from build123d import *

# Parameters (mm, degrees)
SKETCH1_R           = 6.35
BOSS_EXTRUDE1_DEPTH = 31.75
CUT_EXTRUDE1_DEPTH  = 19.05
SKETCH3_R           = 3.175
CUT_EXTRUDE2_DEPTH  = 12.7


with BuildPart() as part:
    # Sketch1 → Boss-Extrude1 (new body)
    with BuildSketch(Plane.XY):
        Circle(SKETCH1_R)
    extrude(amount=BOSS_EXTRUDE1_DEPTH)

    # Sketch2 → Cut-Extrude1 (cut)
    with BuildSketch(Plane.XY.offset(31.75)):
        with BuildLine():
            Line((2.016062499, 2.286), (-2.016062499, 2.286))
            ThreePointArc((-2.016062499, 2.286), (0, -3.048), (2.016062499, 2.286))
        make_face()
    extrude(amount=-CUT_EXTRUDE1_DEPTH, mode=Mode.SUBTRACT)

    # Sketch3 → Cut-Extrude2 (cut)
    with BuildSketch(Plane(origin=(0, 0, 0), x_dir=(-1, 0, 0), z_dir=(0, 0, -1))):
        Circle(SKETCH3_R)
    extrude(amount=-CUT_EXTRUDE2_DEPTH, mode=Mode.SUBTRACT)


solid = part.part
Input: part model. Units: mm. Frame: model coordinates. A direction names the side the tool comes from. Give positions to 0.01 mm unless a question says otherwise; leave off trailing zeros. Order: outer loops, then holes, each group sorted by start corner. A loop starts at its lowest first (then second) coordinate and runs counter-clockwise, first axis right, second up. Notation, with made-up numbers: (-1.75, 60.25) -> (56.25, 60.25) arc R13 cw to (56.25, 73.25) -> close; hole circle Ø3 at (76, 48.5). An arc over 180 degrees is marked (long way). Use one line per item in the form item = value.
1) First-contact query: pin 1 Ø1.5 at (y, z) = (5, 24.5) entering from -X; pin 2 Ø1 at (y, z) = (-4, 20) entering from -X; pin 3 Ø5 at (y, z) = (3, 5.5) entering from -X; pin 4 Ø3.5 at (x, y) = (0, 0) entering from +Z. Flat tips, straight axial feed; report the tip coordinate or a pass-through.
Response values:
pin_1 = -4.72
pin_2 = -5.3
pin_3 = -6.33
pin_4 = through
2) Section D-D, the plane x = 4. Return loops of the section in (y, z).
Response values:
outline = (-4.93, 0) -> (4.93, 0) -> (4.93, 31.75) -> (-4.93, 31.75) -> close
3) Section A-A, the plane x = 0. Return loops of the section in (y, z) (3 decimals), and give its area (3 significant figures).
Response values:
outline = (-6.35, 0) -> (-3.175, 0) -> (-3.175, 12.7) -> (-3.048, 12.7) -> (-3.048, 31.75) -> (-6.35, 31.75) -> close; (2.286, 12.7) -> (3.175, 12.7) -> (3.175, 0) -> (6.35, 0) -> (6.35, 31.75) -> (2.286, 31.75) -> close
area = 221 mm^2
4) Mould query, pull axis Y, two halves, no side actions, for faces 1 (the cylindrical face through (-1.38, -6.2, 15.65)), 2 (the cylindrical face through (0.69, -3.1, 6.26)), 3 (the flat face through (-2, 3, 0)). Classes: pulls with the +Y half, pulls with the -Y half, needs draft (parallel to the pull), parting line crosses it, or undercut.
Response values:
face_1 = parting line crosses it
face_2 = undercut
face_3 = needs draft
5) Section C-C, the plane z = 17.5. Return loops of the section in (x, y).
Response values:
outline = circle Ø12.7 at (0, 0); hole (-2.02, 2.29) arc R3.05 ccw (long way) to (2.02, 2.29) -> close
6) Section B-B, the plane y = 0. Return loops of the section in (x, z) (3 decimals).
Response values:
outline = (-6.35, 0) -> (-3.175, 0) -> (-3.175, 12.7) -> (-3.048, 12.7) -> (-3.048, 31.75) -> (-6.35, 31.75) -> close; (3.048, 12.7) -> (3.175, 12.7) -> (3.175, 0) -> (6.35, 0) -> (6.35, 31.75) -> (3.048, 31.75) -> close
7) Line query: probe 1 along Y at (x, z) = (0, 9.75) (3 decimals); probe 2 along Y at (x, z) = (1.5, 13.5); probe 3 along Z at (x, y) = (0.5, 2.75). Output: solid intervals per line, ascending.
Response values:
probe_1 = -6.35 to -3.175, 3.175 to 6.35
probe_2 = -6.17 to -2.65, 2.29 to 6.17
probe_3 = 12.7 to 31.75
8) Reachability of faces 4 (the flat face through (0, 3, 31.75)), 5 (the flat face through (0, 2.286, 22)) from +Z, -Z, +X, -X, +Y, -Y: full face, straight path, thin tool, end or side. Return the list, or none.
Response values:
face_4 = +Z, +X, -X, +Y, -Y
face_5 = +Z, -Z
